```python
from build123d import *

# Parameters (mm, degrees)
SKETCH1_R           = 50
BOSS_EXTRUDE1_DEPTH = 3
SKETCH3_W           = 40
SKETCH3_H           = 3
BOSS_EXTRUDE3_DEPTH = 60
SKETCH4_R           = 1.5
BOSS_EXTRUDE4_DEPTH = 63
FILLET1_R           = 10


with BuildPart() as part:
    # Sketch1 → Boss-Extrude1 (new body)
    with BuildSketch(Plane(origin=(0, 0, 0), x_dir=(1, 0, 0), z_dir=(0, 1, 0))):
        with Locations(Location((0, 0, 0), (0, 0, 270))):
            Circle(SKETCH1_R)
    extrude(amount=BOSS_EXTRUDE1_DEPTH)

    # Sketch3 → Boss-Extrude3 (add)
    with BuildSketch(Plane(origin=(0, 3, 0), x_dir=(1, 0, 0), z_dir=(0, 1, 0))):
        with Locations((0, -31.5)):
            Rectangle(SKETCH3_W, SKETCH3_H)
        with Locations((0, 31.5)):
            Rectangle(SKETCH3_W, SKETCH3_H)
    extrude(amount=BOSS_EXTRUDE3_DEPTH)

    # Sketch4 → Boss-Extrude4 (add)
    with BuildSketch(Plane.XY.offset(33)):
        with Locations((0, 53)):
            Circle(SKETCH4_R)
        with Locations((0, 15.5)):
            Circle(SKETCH4_R)
    extrude(amount=-BOSS_EXTRUDE4_DEPTH)

    # Fillet1
    fillet1_edges = [part.edges().sort_by_distance(p)[0] for p in [
        (-20, 63, -31.5),
        (20, 63, -31.5),
        (-20, 63, 31.5),
        (20, 63, 31.5),
    ]]
    fillet(fillet1_edges, radius=FILLET1_R)


solid = part.part
```
CAD build for the part. Positions are in the model's coordinates, mm. A direction names the side the tool comes from. Round coordinates to 2 decimals unless told otherwise and drop trailing zeros. Loops run counter-clockwise (first coordinate to the right, second up) from the corner with the lowest first, then second, coordinate; pieces in that order, holes last. Notation, with made-up numbers: (-11, 24) - (36, 24) arc R5 cw to (36, 29) - close; hole circle Ø10 at (-21.75, 26.25). An arc over 180 degrees is marked (long way). Return JSON: item names as keys, results as strings. Group by question number.
Q1. Band-saw the part on B-B on y = 37.5. Give the cut face in (x, z), plus the area to 3 significant figures.
Q2. Tool access for faces 4 (the face through (-1.11, 16.51, 0.42)), 5 (the face through (0, 33, 33)), 6 (the face through (0, 33, -33)), 7 (the face through (20, 28, -31)): list every direction of +Z, -Z, +X, -X, +Y, -Y with a clear straight run to the whole face (end or side of a thin tool).
Q3. Band-saw the part on D-D on y = 15.5. Give the cut face in (x, z), plus the area to 3 significant figures.
Q4. Band-saw the part on A-A on z = 0. Give the cut face in (x, y).
Q5. Flat gauge pins, fed straight in: pin 1 Ø0.9 at (y, z) = (37.5, 31) entering from -X; pin 2 Ø20 at (x, y) = (2.5, 48) entering from +Z; pin 3 Ø20 at (x, y) = (2, 29.5) entering from -Z. Where does each tip first touch, or does it go through?
Q6. Band-saw the part on C-C on x = 0. Give the cut face in (y, z).
Q7. Two-plate mould, pull along Y, no slides. Class faces 1 (the face through (-0.325, 51.536, 0.42)), 2 (the face through (-20, 28, -31)), 3 (the face through (0, 63, 31)): +Y half, -Y half, draft (parallel to the pull), parting line (faces both ways), or undercut.
Q8. Drill centre lines: line 1 along Z through (x, y) = (2.5, 4); line 2 along Y through (x, z) = (-5, 41); line 3 along X through (y, z) = (40, -31.5). Where is each one in solid material? Low to high. Write a range as [from, to].
Solutions:
{
 "1": {"outline": "(-20, -33) - (20, -33) - (20, -30) - (-20, -30) - close; (-20, 30) - (20, 30) - (20, 33) - (-20, 33) - close", "area": "240 mm^2"},
 "2": {"face 4": "none", "face 5": "+Z, +X, -X, +Y", "face 6": "-Z, +X, -X, +Y", "face 7": "+Z, -Z, +X, +Y"},
 "3": {"outline": "(-20, -33) - (20, -33) - (20, -30) - (1.5, -30) - (1.5, 30) - (20, 30) - (20, 33) - (-20, 33) - (-20, 30) - (-1.5, 30) - (-1.5, -30) - (-20, -30) - close", "area": "420 mm^2"},
 "4": {"outline": "(-50, 0) - (50, 0) - (50, 3) - (-50, 3) - close; circle Ø3 at (0, 15.5); circle Ø3 at (0, 53)"},
 "5": {"pin 1": "stops at x = -20", "pin 2": "stops at z = 33", "pin 3": "stops at z = -33"},
 "6": {"outline": "(0, -50) - (3, -50) - (3, -33) - (63, -33) - (63, -30) - (54.5, -30) - (54.5, 30) - (63, 30) - (63, 33) - (3, 33) - (3, 50) - (0, 50) - close; hole (3, -30) - (14, -30) - (14, 30) - (3, 30) - close; hole (17, -30) - (51.5, -30) - (51.5, 30) - (17, 30) - close"},
 "7": {"face 1": "undercut", "face 2": "draft", "face 3": "+Y half"},
 "8": {"line 1": "z = [-33, -30], [30, 33]", "line 2": "y = [0, 3]", "line 3": "x = [-20, 20]"}
}
